Autodesk Inventor part; units mm, degrees
ref_plane "YZ Plane" through (0, 0, 0) normal (1, 0, 0) x (0, 1, 0)
ref_plane "XZ Plane" through (0, 0, 0) normal (0, 1, 0) x (-1, 0, 0)
ref_plane "XY Plane" through (0, 0, 0) normal (0, 0, 1) x (1, 0, 0)
sketch "Sketch1" plane through (0, 0, 0) normal (0, 1, 0) x (-1, 0, 0)
  line L0 (0, 0) -> (-38.1, 0)
  line L1 (-38.1, 0) -> (-38.1, -88.9)
  line L2 (-38.1, -88.9) -> (0, -88.9)
  line L3 (0, -88.9) -> (0, 0)
  dimension "d0" = 38.1
  dimension "d1" = 88.9
extrude "Extrusion1" add sketch "Sketch1" along normal blind 31.75 draft -2
fillet "Fillet1" radius 6.35 4 edges at (0.5544, 15.875, -0.5544) (37.5456, 15.875, -88.3456) (0.5544, 15.875, -88.3456) (37.5456, 15.875, -0.5544)
fillet "Fillet2" radius 0.635 16 edges at (35.133, 31.75, -2.967) (19.05, 31.75, -1.1087) (2.967, 31.75, -2.967) (1.1087, 31.75, -44.45) (2.967, 31.75, -85.933) (19.05, 31.75, -87.7913) (35.133, 31.75, -85.933) (36.9913, 31.75, -44.45) (36.2417, 0, -87.0417) (19.05, 0, -88.9) (1.8583, 0, -87.0417) (0, 0, -44.45) (1.8583, 0, -1.8583) (19.05, 0, 0) (36.2417, 0, -1.8583) (38.1, 0, -44.45)
properties part number "Drive" material "Steel, Cast"
Geometry check sheet. Reference: the model listing, model coordinates, mm. Give positions to 0.01 mm unless a question says otherwise; leave off trailing zeros. Write each loop counter-clockwise with the first axis right and the second up, starting at its lowest first coordinate (ties: lowest second). Pieces come first, ordered by that corner, then holes.
1) Gauge pin test, flat ends, axial feed: pin 1 (8 mm diameter, centred on x = 7, y = 24.5, fed in from -Z); pin 2 (3 mm diameter, centred on y = 28.5, z = -23, fed in from -X); pin 3 (1 mm diameter, centred on y = 15.5, z = -58, fed in from +X); pin 4 (5 mm diameter, centred on x = 11.5, z = -24, fed in from -Y). Record the tip position at first contact, or that the pin passes through.
2) Section check A-A, the plane z = -45. Record the boundary of the cut face in (x, y) (3 decimals).
3) Material ranges on L1, parallel to Z at x = 3, y = 2; L2, parallel to X at y = 20, z = -45; L3, parallel to Z at x = 12.5, y = 4, recorded low to high.
Computed:
1. pin 1: stops at z = -88.18
1. pin 2: stops at x = 0.94
1. pin 3: stops at x = 37.58
1. pin 4: stops at y = 0
2. outline: (0.023, 0.657) arc R0.635 ccw to (0.658, 0) - (37.442, 0) arc R0.635 ccw to (38.077, 0.657) - (37.013, 31.137) arc R0.635 ccw to (36.378, 31.75) - (1.722, 31.75) arc R0.635 ccw to (1.087, 31.137) - close
3. L1: z = -87.83 to -1.07
3. L2: x = 0.7 to 37.4
3. L3: z = -88.76 to -0.14
